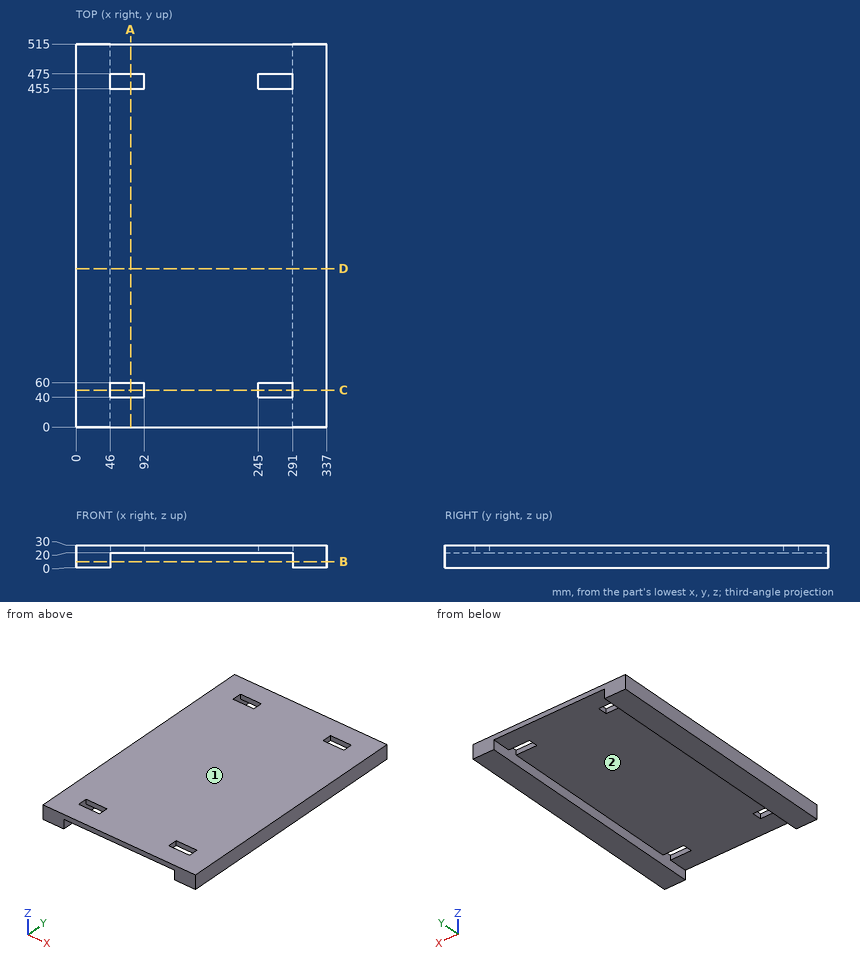
Can you work these out from the drawing? Everything is in mm from the part's minimum corner. Round coordinates to 2 decimals unless told otherwise and drop trailing zeros. Loops run counter-clockwise (first coordinate to the right, second up) from the corner with the lowest first, then second, coordinate; pieces in that order, holes last. Notation, with made-up numbers: M -6.75,89.5 L 17.25,89.5 A13 cw 17.25,114.5 Z; hole C 79,-35 d6. An arc over 180 degrees is marked long. Write item = value, one per line.
1. I want a section at C-C, the plane y = 50. Write out the boundary of the cut face in (x, z).
Results below:
outline = M 0,0 L 46,0 L 46,30 L 0,30 Z; M 92,20 L 245,20 L 245,30 L 92,30 Z; M 291,0 L 337,0 L 337,30 L 291,30 Z
2. I want a section at B-B, the plane z = 8. Write out the boundary of the cut face in (x, y), and give its area (3 significant figures).
Results below:
outline = M 0,0 L 46,0 L 46,515 L 0,515 Z; M 291,0 L 337,0 L 337,515 L 291,515 Z
area = 47,400 mm²
3. Will these pins go through, and if not, where does the flat tip stop? P1, Ø1.5, axis at x = 92, z = 17.5, coming from the -Y side; P2, Ø4, axis at x = 281.5, y = 249, coming from the -Z side.
Results below:
P1 = through
P2 = 20
4. Thinking about a two-plate mould opening in X: for the marked faces 1 and 2, which applies, +X half, -X half, draft (parallel to the pull), parting line (faces both ways), or undercut?
Results below:
face_1 = draft
face_2 = undercut
5. I want a section at D-D, the plane y = 213. Write out the boundary of the cut face in (x, z).
Results below:
outline = M 0,0 L 46,0 L 46,20 L 291,20 L 291,0 L 337,0 L 337,30 L 0,30 Z
6. I want a section at A-A, the plane x = 73.5. Write out the boundary of the cut face in (y, z), and give its area (3 significant figures).
Results below:
outline = M 0,20 L 40,20 L 40,30 L 0,30 Z; M 60,20 L 455,20 L 455,30 L 60,30 Z; M 475,20 L 515,20 L 515,30 L 475,30 Z
area = 4,750 mm²
7. I need wall thicknesses on probe 1 along X at (y, z) = (398.5, 4.25); probe 2 along Z at (x, y) = (159, 119). Which ranges of each line are inside material? Lowest first, please.
Results below:
probe_1 = 0 to 46, 291 to 337
probe_2 = 20 to 30
